from build123d import *

# Parameters (mm, degrees)
BOSS_EXTRUDE1_DEPTH = 14
BOSS_EXTRUDE2_DEPTH = 22.5
CUT_EXTRUDE1_DEPTH  = 67.289139382
SKETCH4_R           = 5
CUT_EXTRUDE2_DEPTH  = 48.86961458


with BuildPart() as part:
    # Sketch1 → Boss-Extrude1 (new, symmetric)
    with BuildSketch(Plane.XY):
        Polygon((-25.5, 39), (-25.5, 0), (25.5, 0), (25.5, 39), (23.5, 39), (23.5, 2), (-23.5, 2), (-23.5, 39), align=None)
    extrude(amount=BOSS_EXTRUDE1_DEPTH, both=True)

    # Sketch2 → Boss-Extrude2 (add, symmetric)
    with BuildSketch(Plane(origin=(0, 0, 0), x_dir=(0, 0, -1), z_dir=(1, 0, 0))):
        Polygon((-14, 0), (-16.5, 0), (-16.5, 7), (-14.5, 7), (-14.5, 2), (-14, 2), align=None)
    boss_extrude2 = extrude(amount=BOSS_EXTRUDE2_DEPTH, both=True)

    # Mirror1: Boss-Extrude2 across plane
    add(boss_extrude2.mirror(Plane.XY))

    # Sketch3 → Cut-Extrude1 (cut, through all)
    with BuildSketch(Plane(origin=(25.5, 0, 0), x_dir=(0, 0, -1), z_dir=(1, 0, 0))):
        with BuildLine():
            Line((-5, 36), (-5, 39))
            Line((-5, 39), (5, 39))
            Line((5, 39), (5, 36))
            ThreePointArc((5, 36), (0, 31), (-5, 36))
        make_face()
    extrude(amount=-CUT_EXTRUDE1_DEPTH, mode=Mode.SUBTRACT)

    # Sketch4 → Cut-Extrude2 (cut, through all)
    with BuildSketch(Plane(origin=(0, 2, 0), x_dir=(1, 0, 0), z_dir=(0, 1, 0))):
        with Locations(Location((0, 0, 0), (0, 0, 270))):
            Circle(SKETCH4_R)
    extrude(amount=-CUT_EXTRUDE2_DEPTH, mode=Mode.SUBTRACT)


solid = part.part
CAD build for the part. Positions are in the model's coordinates, mm. A direction names the side the tool comes from. Round coordinates to 2 decimals unless told otherwise and drop trailing zeros. Order: outer loops, then holes, each group sorted by start corner. A loop starts at its lowest first (then second) coordinate and runs counter-clockwise, first axis right, second up. Notation, with made-up numbers: (-21.5, 37.5) -> (15.5, 37.5) arc R12 ccw to (15.5, 45.5) -> close; hole circle Ø7 at (87, 39.5). An arc over 180 degrees is marked (long way). Write each question's results on one line, items separated by ' | '.
1. Cut at B-B (y = 17.5). Give the cut face in (x, z), plus the area to 3 significant figures.
Findings below:
outline: (-25.5, -14) -> (-23.5, -14) -> (-23.5, 14) -> (-25.5, 14) -> close; (23.5, -14) -> (25.5, -14) -> (25.5, 14) -> (23.5, 14) -> close | area: 112 mm²
2. Pull direction Z, two halves, no side cores. Call faces 4 (the face through (25, 38, -5)), 5 (the face through (-25, 20, -14)), 6 (the face through (25, 39, 10)), 7 (the face through (-24, 37, 5)): pulls with the +Z half, pulls with the -Z half, needs draft (parallel to the pull), parting line crosses it, or undercut.
Findings below:
face 4: undercut | face 5: pulls with the -Z half | face 6: needs draft | face 7: undercut
3. 3-axis set-ups, long thin cutter, end or side, ignore diameter. For faces 1 (the face through (0, 5, 14.5)), 2 (the face through (-22.5, 4, -16)), 3 (the face through (23.5, 21, 0)): which of +Z, -Z, +X, -X, +Y, -Y reach the whole face in a straight line?
Findings below:
face 1: +X, -X, +Y | face 2: -Z, -X, +Y, -Y | face 3: +Z, -Z, +Y
4. Flat gauge pins, fed straight in: P1, Ø0.8, axis at y = 4, z = 15.5, coming from the -X side; P2, Ø1, axis at x = 24.5, y = 38, coming from the +Z side; P3, Ø1, axis at x = -7.5, z = -15.5, coming from the +Y side; P4, Ø1, axis at x = -14, z = 11.5, coming from the -Y side. Where does each tip first touch, or does it go through?
Findings below:
P1: stops at x = -22.5 | P2: stops at z = 14 | P3: stops at y = 7 | P4: stops at y = 0
5. Cut at C-C (x = 0). Give the cut face in (y, z), plus the area to 3 significant figures.
Findings below:
outline: (0, -16.5) -> (7, -16.5) -> (7, -14.5) -> (2, -14.5) -> (2, -5) -> (0, -5) -> close; (0, 5) -> (2, 5) -> (2, 14.5) -> (7, 14.5) -> (7, 16.5) -> (0, 16.5) -> close | area: 66.0 mm²
6. Wall check: line 1 along X through (y, z) = (1.1, 0); line 2 along X through (y, z) = (18, -7); line 3 along Z through (x, y) = (-6.5, 4.5). Give the ranges that are in metal, low to high. Write a range as [from, to].
Findings below:
line 1: x = [-25.5, -5], [5, 25.5] | line 2: x = [-25.5, -23.5], [23.5, 25.5] | line 3: z = [-16.5, -14.5], [14.5, 16.5]
7. Cut at A-A (z = 0). Give the cut face in (x, y), plus the area to 3 significant figures.
Findings below:
outline: (-25.5, 0) -> (-5, 0) -> (-5, 2) -> (-23.5, 2) -> (-23.5, 31) -> (-25.5, 31) -> close; (5, 0) -> (25.5, 0) -> (25.5, 31) -> (23.5, 31) -> (23.5, 2) -> (5, 2) -> close | area: 198 mm²
8. Cut at D-D (x = 10.5). Give the cut face in (y, z), plus the area to 3 significant figures.
Findings below:
outline: (0, -16.5) -> (7, -16.5) -> (7, -14.5) -> (2, -14.5) -> (2, 14.5) -> (7, 14.5) -> (7, 16.5) -> (0, 16.5) -> close | area: 86.0 mm²
